Work out the finished part from the listing and answer in its coordinate system (mm). A direction names the side the tool comes from. Round coordinates to 2 decimals unless told otherwise and drop trailing zeros. Write each loop counter-clockwise with the first axis right and the second up, starting at its lowest first coordinate (ties: lowest second). Pieces come first, ordered by that corner, then holes. Notation, with made-up numbers: (49, -6) -> (98, -6) arc R9 cw to (98, 2) -> close; hole circle Ø9 at (8.25, 7). An arc over 180 degrees is marked (long way). One line per item, written item: value.
```python
from build123d import *

# Parameters (mm, degrees)
SKETCH_W        = 70
SKETCH_H        = 55
PAD_DEPTH       = 22
SKETCH001_R     = 17
POCKET_DEPTH    = 55.001
SKETCH002_R     = 1.53
SKETCH002_W     = 3
SKETCH002_H     = 10
POCKET001_DEPTH = 205.4022
SKETCH003_R     = 4
POCKET002_DEPTH = 7


with BuildPart() as part:
    # Sketch → Pad (new body)
    with BuildSketch(Plane.XY):
        with Locations((0, -17.338946)):
            Rectangle(SKETCH_W, SKETCH_H)
    extrude(amount=PAD_DEPTH)

    # Sketch001 (on Face3 of Pad) → Pocket (cut, through all)
    with BuildSketch(Plane.XZ.offset(44.838946)):
        Circle(SKETCH001_R)
    extrude(amount=-POCKET_DEPTH, mode=Mode.SUBTRACT)

    # Sketch002 (on Face2 of Pocket) → Pocket001 (cut, through all)
    with BuildSketch(Plane(origin=(0, 0, 0), x_dir=(1, 0, 0), z_dir=(0, 0, -1))):
        with Locations((-26.352302, 17.193167)):
            Circle(SKETCH002_R)
        with Locations((-21.951078, -2.806833)):
            Rectangle(SKETCH002_W, SKETCH002_H)
        with Locations((-21.951078, 37.193167)):
            Rectangle(SKETCH002_W, SKETCH002_H)
    pocket001 = extrude(amount=-POCKET001_DEPTH, mode=Mode.SUBTRACT)

    # Mirrored: Pocket001 across Sketch002 V_Axis
    add(pocket001.mirror(Plane(origin=(0, 0, 0), x_dir=(0, 0, -1), z_dir=(1, 0, 0))), mode=Mode.SUBTRACT)

    # Sketch003 (on Face2 of Mirrored) → Pocket002 (cut)
    with BuildSketch(Plane(origin=(0, 0, 0), x_dir=(1, 0, 0), z_dir=(0, 0, -1))):
        with Locations((-26.352302, 17.193167)):
            Circle(SKETCH003_R)
    pocket002 = extrude(amount=-POCKET002_DEPTH, mode=Mode.SUBTRACT)

    # Mirrored001: Pocket002 across Sketch003 V_Axis
    add(pocket002.mirror(Plane(origin=(0, 0, 0), x_dir=(0, 0, -1), z_dir=(1, 0, 0))), mode=Mode.SUBTRACT)


solid = part.part
```
(1) Find section D-D on x = 0. Give the vertices of the cut face in (y, z), plus the area to 3 significant figures.
Reported:
outline: (-44.84, 17) -> (10.16, 17) -> (10.16, 22) -> (-44.84, 22) -> close
area: 275 mm2
(2) Find section B-B on y = -8. Give the vertices of the cut face in (x, z), plus the area to 3 significant figures.
Reported:
outline: (-35, 0) -> (-17, 0) arc R17 cw to (17, 0) -> (35, 0) -> (35, 22) -> (-35, 22) -> close
area: 1,090 mm2
(3) For a pull along Y with two mould halves and no side action, classify faces 1 (the face through (-22, -17, 0)), 2 (the face through (-20.451, 3, 11)), 3 (the face through (0, 10.161, 18)) as pulls with the +Y half, pulls with the -Y half, needs draft (parallel to the pull), parting line crosses it, or undercut.
Reported:
face 1: needs draft
face 2: undercut
face 3: pulls with the +Y half
(4) A tool of negligible diameter and unlimited length cuts with its end or side. For faces 4 (the face through (22, -17, 0)), 5 (the face through (-22, -42.193, 11)), 6 (the face through (24.6, -17.2, 7)), from which of +Z, -Z, +X, -X, +Y, -Y can it reach the whole face along a straight path? Write none if from no direction.
Reported:
face 4: -Z, +X, -X, +Y, -Y
face 5: +Z, -Z
face 6: -Z
(5) Find section A-A on z = 16.25. Give the vertices of the cut face in (x, y), plus the area to 3 significant figures.
Reported:
outline: (-35, -44.84) -> (-4.99, -44.84) -> (-4.99, 10.16) -> (-35, 10.16) -> close; (4.99, -44.84) -> (35, -44.84) -> (35, 10.16) -> (4.99, 10.16) -> close; hole circle Ø3.06 at (-26.35, -17.19); hole (-23.45, -42.19) -> (-20.45, -42.19) -> (-20.45, -32.19) -> (-23.45, -32.19) -> close; hole (-23.45, -2.19) -> (-20.45, -2.19) -> (-20.45, 7.81) -> (-23.45, 7.81) -> close; hole (20.45, -42.19) -> (23.45, -42.19) -> (23.45, -32.19) -> (20.45, -32.19) -> close; hole (20.45, -2.19) -> (23.45, -2.19) -> (23.45, 7.81) -> (20.45, 7.81) -> close; hole circle Ø3.06 at (26.35, -17.19)
area: 3,170 mm2
(6) Find section C-C on z = 12. Give the vertices of the cut face in (x, y), plus the area to 3 significant figures.
Reported:
outline: (-35, -44.84) -> (-12.04, -44.84) -> (-12.04, 10.16) -> (-35, 10.16) -> close; (12.04, -44.84) -> (35, -44.84) -> (35, 10.16) -> (12.04, 10.16) -> close; hole circle Ø3.06 at (-26.35, -17.19); hole (-23.45, -42.19) -> (-20.45, -42.19) -> (-20.45, -32.19) -> (-23.45, -32.19) -> close; hole (-23.45, -2.19) -> (-20.45, -2.19) -> (-20.45, 7.81) -> (-23.45, 7.81) -> close; hole (20.45, -42.19) -> (23.45, -42.19) -> (23.45, -32.19) -> (20.45, -32.19) -> close; hole (20.45, -2.19) -> (23.45, -2.19) -> (23.45, 7.81) -> (20.45, 7.81) -> close; hole circle Ø3.06 at (26.35, -17.19)
area: 2,390 mm2
(7) Consider probe 1 along X at (y, z) = (-36.5, 18.25); probe 2 along X at (y, z) = (-20, 2.5); probe 3 along X at (y, z) = (3, 7.75). Determine where each line is inside the solid, lowest interval first.
Reported:
probe 1: x = -35 to -23.45, -20.45 to 20.45, 23.45 to 35
probe 2: x = -35 to -29.2, -23.5 to -16.82, 16.82 to 23.5, 29.2 to 35
probe 3: x = -35 to -23.45, -20.45 to -15.13, 15.13 to 20.45, 23.45 to 35
(8) Flat-ended cylindrical pins translate along their axes: pin 1 Ø6.5 at (x, y) = (26, -17) entering from -Z; pin 2 Ø1 at (x, y) = (11, -38) entering from -Z; pin 3 Ø1 at (x, y) = (13.5, -17) entering from -Z. Find the tip coordinate at first contact, or state that the pin passes through.
Reported:
pin 1: stops at z = 7
pin 2: stops at z = 12.52
pin 3: stops at z = 9.64
